```python
from build123d import *

# Parameters (mm, degrees)
EXTRUDE_1_DEPTH            = 5
FILLET_1_R                 = 2
HOLE_WIZARD_M3_1_OUTLINE_R = 1.7
HOLE_WIZARD_M3_1_DEPTH     = 5
SKETCH_4_R                 = 15
CUT_EXTRUDE_1_DEPTH        = 10
HOLE_WIZARD_M3_5_D         = 3.4


# Read off the part's stored shape, not the designer's step: M3 间隙孔1
with BuildPart() as part:
    # 草图1 → 凸台-拉伸1 (new body)
    with BuildSketch(Plane.XY):
        Polygon((30, 0), (57.5, 31.083095625), (107.5, 31.083095625), (135, 0), (165, 0), (165, 6), (136.367610504, 6), (107.098159975, 39.083095625), (103.5, 39.083095625), (103.5, 75.083095625), (61.5, 75.083095625), (61.5, 39.083095625), (57.901840025, 39.083095625), (28.632389496, 6), (0, 6), (0, 0), align=None)
    extrude(amount=EXTRUDE_1_DEPTH)

    # 圆角1
    fillet_1_edges = [part.edges().sort_by_distance(p)[0] for p in [
        (28.632389496, 6, 2.5),
        (0, 6, 2.5),
        (0, 0, 2.5),
        (30, 0, 2.5),
        (57.5, 31.083095625, 2.5),
        (107.5, 31.083095625, 2.5),
        (135, 0, 2.5),
        (165, 0, 2.5),
        (165, 6, 2.5),
        (136.367610504, 6, 2.5),
        (107.098159975, 39.083095625, 2.5),
        (103.5, 39.083095625, 2.5),
        (103.5, 75.083095625, 2.5),
        (61.5, 75.083095625, 2.5),
        (61.5, 39.083095625, 2.5),
        (57.901840025, 39.083095625, 2.5),
    ]]
    fillet(fillet_1_edges, radius=FILLET_1_R)

    # M3 间隙孔1 outline → M3 间隙孔1 (cut)
    with BuildSketch(Plane.XY):
        with Locations((98, 69.583095625)):
            Circle(HOLE_WIZARD_M3_1_OUTLINE_R)
        with Locations((67, 38.583095625)):
            Circle(HOLE_WIZARD_M3_1_OUTLINE_R)
        with Locations((98, 38.583095625)):
            Circle(HOLE_WIZARD_M3_1_OUTLINE_R)
        with Locations((67, 69.583095625)):
            Circle(HOLE_WIZARD_M3_1_OUTLINE_R)
    extrude(amount=HOLE_WIZARD_M3_1_DEPTH, mode=Mode.SUBTRACT)

    # 草图4 → 切除-拉伸1 (cut)
    with BuildSketch(Plane.XY.offset(5)):
        with Locations((82.5, 54.083095625)):
            Circle(SKETCH_4_R)
    extrude(amount=-CUT_EXTRUDE_1_DEPTH, mode=Mode.SUBTRACT)

    # M3 间隙孔5 (through all)
    with Locations(Plane.XY.offset(5)):
        with Locations((7.5, 3), (157.5, 3)):
            Hole(HOLE_WIZARD_M3_5_D / 2)


solid = part.part
```
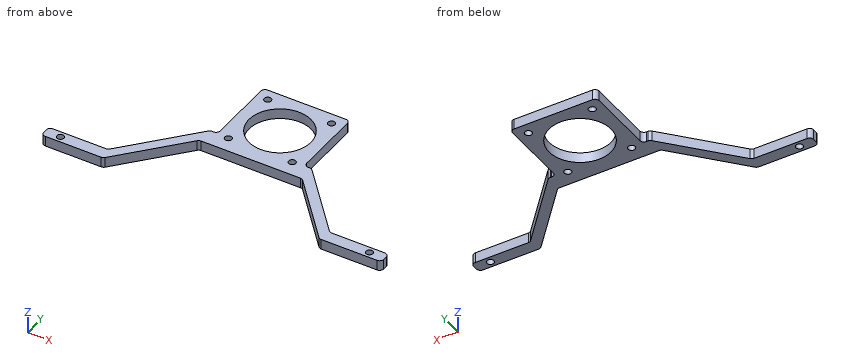
Read the model definition and answer for the solid it produces. Units are mm, in the model's axes. Give positions to 0.01 mm unless a question says otherwise; leave off trailing zeros. Write each loop counter-clockwise with the first axis right and the second up, starting at its lowest first coordinate (ties: lowest second). Pieces come first, ordered by that corner, then holes. Notation, with made-up numbers: M 87,74.25 L 107,74.25 A21 cw 107,100.25 Z; hole C 60,-32 d10. An arc over 180 degrees is marked long. Put each result on its own line as item: value. Start each with the question number.
1. The part is cut by section D-D, the plane z = 2.3. Give the number of separate pieces and of enclosed holes in the cut face, and give its area (3 significant figures).
2. The part is cut by section C-C, the plane x = 117. Give the vertices of the cut face in (y, z), and give its area (3 significant figures).
3. Consider line 1 along Y through (x, z) = (67, 2.75); line 2 along Y through (x, z) = (82.5, 3.3); line 3 along Y through (x, z) = (157.5, 2.1). Determine where each line is inside the solid, lowest interval first.
4. The part is cut by section A-A, the plane x = 157.5. Give the vertices of the cut face in (y, z), and give its area (3 significant figures).
5. The part is cut by section B-B, the plane y = 66. Give the vertices of the cut face in (x, z).
6. Each of these flat-tipped pins is pushed along its axis until it touches: pin 1 Ø0.8 at (x, z) = (106, 1.5) entering from +Y; pin 2 Ø5.5 at (x, y) = (157.5, 3) entering from +Z; pin 3 Ø1.5 at (x, z) = (92.5, 1.5) entering from -Y; pin 4 Ø2.5 at (y, z) = (51.5, 2) entering from +X. Where does it stop, or does it pass through?
Final values:
1. separate pieces: 1
1. enclosed holes: 7
1. area: 1,920 mm²
2. outline: M 20.35,0 L 27.89,0 L 27.89,5 L 20.35,5 Z
2. area: 37.7 mm²
3. line 1: y = 31.08 to 36.88, 40.28 to 67.88, 71.28 to 75.08
3. line 2: y = 31.08 to 39.08, 69.08 to 75.08
3. line 3: y = 0 to 1.3, 4.7 to 6
4. outline: M 0,0 L 1.3,0 L 1.3,5 L 0,5 Z; M 4.7,0 L 6,0 L 6,5 L 4.7,5 Z
4. area: 13.0 mm²
5. outline: M 61.5,0 L 73.39,0 L 73.39,5 L 61.5,5 Z; M 91.61,0 L 103.5,0 L 103.5,5 L 91.61,5 Z
6. pin 1: stops at y = 39.08
6. pin 2: stops at z = 5
6. pin 3: stops at y = 31.08
6. pin 4: stops at x = 103.5
